Can you work these out from the drawing? Everything is in mm from the part's minimum corner. A direction names the side the tool comes from. Coordinates: 2 decimals unless noted, no trailing zeros. Write each loop counter-clockwise with the first axis right and the second up, starting at its lowest first coordinate (ties: lowest second). Pieces come first, ordered by that corner, then holes. Notation, with made-up numbers: M 81.25,43.25 L 93.25,43.25 A17 cw 93.25,53.25 Z; hole C 26.25,41 d9. An arc over 180 degrees is marked long. Write each question's results on one line, items separated by ' | '. Start each with the question number.
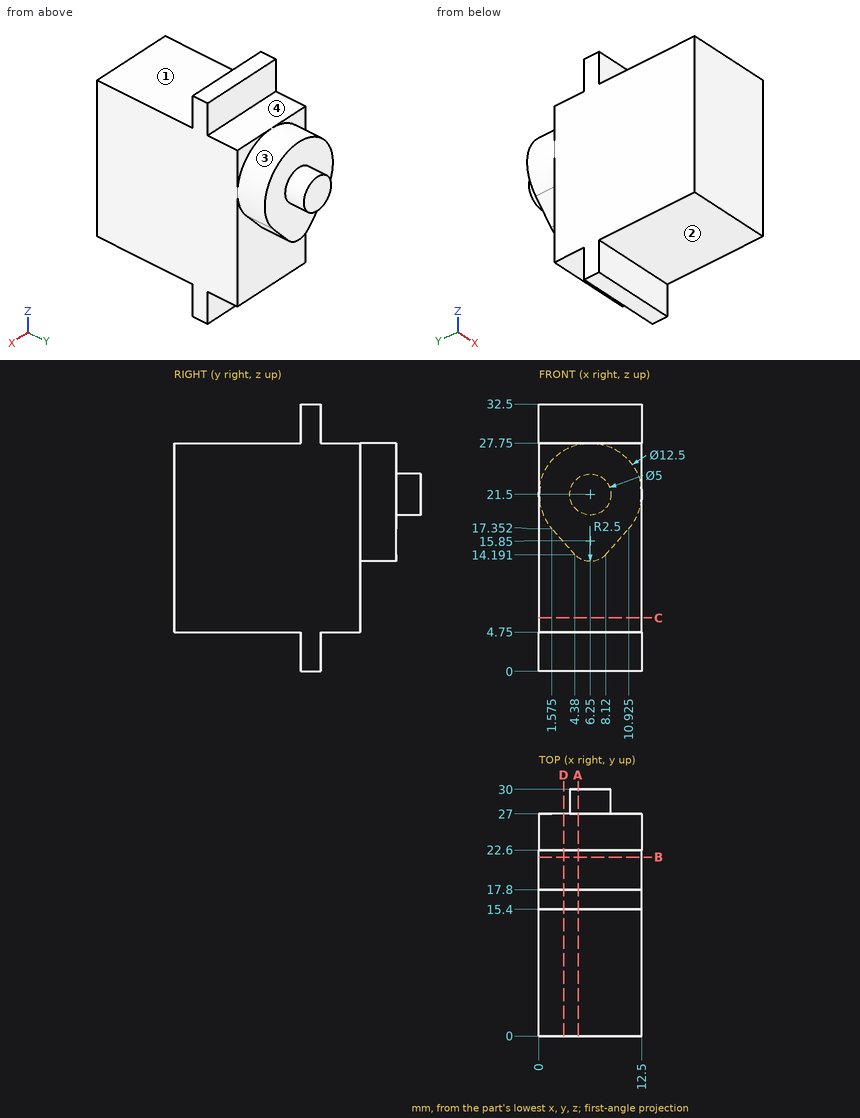
1) I want a section at D-D, the plane x = 3. Write out the boundary of the cut face in (y, z), then the cut area to 3 significant figures.
2) Please list where these lines run through material, in increasing order: line 1 (Z direction, x = 3, y = 10); line 2 (Y direction, x = 2, z = 7.5); line 3 (Y direction, x = 2.5, z = 22). Write a range as [from, to].
3) I want a section at B-B, the plane y = 21.75. Write out the boundary of the cut face in (x, z), then the cut area to 4 significant figures.
4) For pin 1 Ø6 at (x, y) = (3.5, 6) entering from -Z; pin 2 Ø6 at (x, y) = (5.5, 6) entering from +Z; pin 3 Ø1.9 at (x, z) = (10.5, 26) entering from +Y, each with a flat end and sliding along its axis, tell me the tip position at first contact or that it passes through.
5) I want a section at A-A, the plane x = 4.75. Write out the boundary of the cut face in (y, z).
6) For the marked faces 1, 2, 3 and 4, which set-ups out of +Z, -Z, +X, -X, +Y, -Y let a thin tool reach every point of the face, with its end or its side?
7) I want a section at C-C, the plane z = 6.5. Write out the boundary of the cut face in (x, y).
Output:
1) outline: M 0,4.75 L 15.4,4.75 L 15.4,0 L 17.8,0 L 17.8,4.75 L 22.6,4.75 L 22.6,15.75 L 27,15.75 L 27,26.84 L 22.6,26.84 L 22.6,27.75 L 17.8,27.75 L 17.8,32.5 L 15.4,32.5 L 15.4,27.75 L 0,27.75 Z | area: 591 mm2
2) line 1: z = [4.75, 27.75] | line 2: y = [0, 22.6] | line 3: y = [0, 27]
3) outline: M 0,4.75 L 12.5,4.75 L 12.5,27.75 L 0,27.75 Z | area: 287.5 mm2
4) pin 1: stops at z = 4.75 | pin 2: stops at z = 27.75 | pin 3: stops at y = 27
5) outline: M 0,4.75 L 15.4,4.75 L 15.4,0 L 17.8,0 L 17.8,4.75 L 22.6,4.75 L 22.6,13.85 L 27,13.85 L 27,19.5 L 30,19.5 L 30,23.5 L 27,23.5 L 27,27.57 L 22.6,27.57 L 22.6,27.75 L 17.8,27.75 L 17.8,32.5 L 15.4,32.5 L 15.4,27.75 L 0,27.75 Z
6) face 1: +Z, +X, -X, -Y | face 2: -Z, +X, -X, -Y | face 3: +Y | face 4: +Z, +X, -X, +Y
7) outline: M 0,0 L 12.5,0 L 12.5,22.6 L 0,22.6 Z
